Autodesk Inventor part; units mm, degrees
ref_plane "YZ Plane" through (0, 0, 0) normal (1, 0, 0) x (0, 1, 0)
ref_plane "XZ Plane" through (0, 0, 0) normal (0, 1, 0) x (-1, 0, 0)
ref_plane "XY Plane" through (0, 0, 0) normal (0, 0, 1) x (1, 0, 0)
sketch "Sketch1" plane through (0, 0, 0) normal (0, 1, 0) x (-1, 0, 0)
  line L0 (4, 10) -> (-19.4211, 10)
  line L1 (-19.4211, -10) -> (4, -10)
  line L2 (4, -10) -> (4, 10)
  arc A0 (-19.4211, -10) -> (-19.4211, 10) centre (-25.1, 0) ccw
  line L3 (4, -10) -> (6, -10)
  line L4 (6, -10) -> (6, 10)
  line L5 (6, 10) -> (4, 10)
  line L6 (4, 10) -> (4, -10)
  point P0 (0, 0)
  dimension "d0" = 20
  dimension "d2" = 4
  dimension "d3" = 10
  dimension "d6" = 10
  dimension "d7" = 23
  dimension "d8" = 29.1
  dimension "d11" = 23.4211
  dimension "d12" = 20
  dimension "d13" = 2
extrude "Extrusion1" add sketch "Sketch1" along normal blind 7.07
fillet "Fillet1" radius 1 2 edges at (19.4211, 3.535, 10) (19.4211, 3.535, -10)
sketch "Sketch2" plane through (0, 7.07, 0) normal (0, 1, 0) x (1, 0, 0)
  circle A0 centre (0.68, 0) radius 0.7835
  circle A1 centre (7.98, -7) radius 0.7835
  circle A2 centre (7.98, 7) radius 0.7835
  circle A3 centre (0, -8.07) radius 0.7835
  circle A4 centre (0, 8.07) radius 0.7835
  circle A5 centre (-3, 8.07) radius 1.05
  circle A6 centre (4.98, 7) radius 1.05
  circle A7 centre (-2.32, 0) radius 1.05
  circle A8 centre (4.98, -7) radius 1.05
  circle A9 centre (-3, -8.07) radius 1.05
  point P0 (0, 0)
hole "Hole1" at (4.98, 7.07, 7) at (-2.32, 7.07, 0) at (-3, 7.07, 8.07) at (-3, 7.07, -8.07) at (4.98, 7.07, -7) direction (0, -1, 0) diameter 2.1 depth 7.07
sketch "Sketch3" plane through (0, 0, 0) normal (0, -1, 0) x (1, 0, 0)
  line L0 (18.1137, 10.8993) -> (3.779, -13.929)
  arc A0 (17.1193, 8.28) -> (17.1193, -8.28) centre (25.1, 0) ccw
  line L1 (16.4253, -10) -> (-6, -10)
  arc A1 (16.4253, -10) -> (17.1193, -8.28) centre (16.4253, -9) ccw
  point P0 (0, 0)
  point P1 (15.1407, 5.75)
  point P2 (6.0474, -10)
  dimension "d22" = 60
extrude "Extrusion2" cut sketch "Sketch3" against normal up to next
properties part number "3D_printed_part"
Part model, mm, in its own coordinate system. Give positions to 0.01 mm unless a question says otherwise; leave off trailing zeros. Loops run counter-clockwise (first coordinate to the right, second up) from the corner with the lowest first, then second, coordinate; pieces in that order, holes last.
(1) Pin check, flat tip, straight feed: pin 1 (1.9 mm diameter, centred on x = -3, z = 8.07, fed in from +Y). Stop position of the tip, or through.
Return value:
pin 1: passes through
(2) Drill centre lines: line 1 along Z through (x, y) = (5, 6.75); line 2 along Z through (x, y) = (-3, 2.75); line 3 along Z through (x, y) = (5.5, 2.25). Where is each one in solid material? Low to high.
Return value:
line 1: z = -10 to -8.05, -5.95 to 5.95, 8.05 to 10
line 2: z = -10 to -9.12, -7.02 to -0.8, 0.8 to 7.02, 9.12 to 10
line 3: z = -10 to -7.91, -6.09 to 6.09, 7.91 to 10
(3) Pull direction X, two halves, no side cores. Call faces 1 (the flat face through (10.66, 3.49, -2.01)), 2 (the cylindrical face through (6.005, 3.486, -7.228)), 3 (the flat face through (-6, 3, 0)), 4 (the flat face through (3, 0, 2)): pulls with the +X half, pulls with the -X half, needs draft (parallel to the pull), parting line crosses it, or undercut.
Return value:
face 1: pulls with the +X half
face 2: undercut
face 3: pulls with the -X half
face 4: needs draft
(4) Band-saw the part on A-A (y = 5). Write the cut outline in (x, z), and give its area (3 significant figures).
Return value:
outline: (-6, -10) - (6.05, -10) - (15.14, 5.75) arc R11.5 cw to (17.12, 8.28) arc R1 ccw to (16.43, 10) - (-6, 10) - close; hole circle Ø2.1 at (-3, -8.07); hole circle Ø2.1 at (-3, 8.07); hole circle Ø2.1 at (-2.32, 0); hole circle Ø2.1 at (4.98, -7); hole circle Ø2.1 at (4.98, 7)
area: 340 mm2
(5) Band-saw the part on B-B (x = 4.98). Write the cut outline in (y, z).
Return value:
outline: (0, -10) - (7.07, -10) - (7.07, -8.05) - (0, -8.05) - close; (0, -5.95) - (7.07, -5.95) - (7.07, 5.95) - (0, 5.95) - close; (0, 8.05) - (7.07, 8.05) - (7.07, 10) - (0, 10) - close
(6) Band-saw the part on D-D (z = 0.5). Write the cut outline in (x, y).
Return value:
outline: (-6, 0) - (-3.24, 0) - (-3.24, 7.07) - (-6, 7.07) - close; (-1.4, 0) - (12.11, 0) - (12.11, 7.07) - (-1.4, 7.07) - close
(7) Band-saw the part on C-C (x = -2.32). Write the cut outline in (y, z), and give its area (3 significant figures).
Return value:
outline: (0, -10) - (7.07, -10) - (7.07, -8.87) - (0, -8.87) - close; (0, -7.27) - (7.07, -7.27) - (7.07, -1.05) - (0, -1.05) - close; (0, 1.05) - (7.07, 1.05) - (7.07, 7.27) - (0, 7.27) - close; (0, 8.87) - (7.07, 8.87) - (7.07, 10) - (0, 10) - close
area: 104 mm2
